Part model, mm, in its own coordinate system. Face numbers are marked on the shaded views. Coordinates: 2 decimals unless noted, no trailing zeros. Loops run counter-clockwise (first coordinate to the right, second up) from the corner with the lowest first, then second, coordinate; pieces in that order, holes last. Notation, with made-up numbers: (36, 10.5) - (44, 10.5) arc R14 ccw to (44, 25.5) - close; hole circle Ø11 at (-19, 80). An arc over 180 degrees is marked (long way). Use a Markdown table: item, result. Add a question column.
1. Band-saw the part on C-C, the plane x = 15.5. Give the cut face in (y, z).
2. Drop flat-ended pins along their axis: pin 1 (4 mm diameter, centred on x = 0, y = -9.5, fed in from -Z); pin 2 (5.5 mm diameter, centred on x = -15.5, y = 0, fed in from +Z); pin 3 (2 mm diameter, centred on x = -7.5, z = 2, fed in from +Y); pin 4 (1.5 mm diameter, centred on x = -5.5, z = 3, fed in from -Y). Give the stop position or say it passes through.
3. Band-saw the part on D-D, the plane x = -11. Give the cut face in (y, z).
4. Band-saw the part on B-B, the plane y = 0. Give the cut face in (x, z), plus the area to 3 significant figures.
5. Wall check: probe 1 along Y at (x, z) = (0, 1.2); probe 2 along Y at (x, z) = (0, 3.4); probe 3 along Z at (x, y) = (14, -1.5). Give the ranges that are in metal, low to high. Write a range as [from, to].
6. Pull direction X, two halves, no side cores. Call the marked faces 1, 2 and 3: pulls with the +X half, pulls with the -X half, needs draft (parallel to the pull), parting line crosses it, or undercut.
7. Band-saw the part on A-A, the plane z = 3.8. Give the cut face in (x, y), plus the area to 3 significant figures.
from build123d import *

# Parameters (mm, degrees)
F0_R     = 22.5
F1_DEPTH = 5
F3_DEPTH = 25
F5_DEPTH = 25
F6_R     = 2
F7_DEPTH = 25
F8_R     = 3.5
F9_DEPTH = 2.5


with BuildPart() as f1:
    # F0 (on Top) → F1 (new body)
    with BuildSketch(Plane.XY):
        Circle(F0_R)
    extrude(amount=F1_DEPTH)

    # F2 (on face) → F3 (cut)
    with BuildSketch(Plane.XY.offset(5)):
        with BuildLine():
            Line((2.7, 0), (2.7, 2.5298221281))
            ThreePointArc((2.7, 2.5298221281), (-3.7, 0), (2.7, -2.5298221281))
            Line((2.7, -2.5298221281), (2.7, 0))
        make_face()
    extrude(amount=-F3_DEPTH, mode=Mode.SUBTRACT)

    # F4 (on face) → F5 (cut)
    with BuildSketch(Plane.XY.offset(5)):
        with BuildLine():
            ThreePointArc((0, 17.5), (-1.4142135624, 14.0857864376), (2, 15.5))
            ThreePointArc((2, 15.5), (1.4142135624, 16.9142135624), (0, 17.5))
        make_face()
    extrude(amount=-F5_DEPTH, mode=Mode.SUBTRACT)

    # F6 (on face) → F7 (cut)
    with BuildSketch(Plane.XY.offset(5)):
        with Locations((15.5, 0)):
            Circle(F6_R)
        with BuildLine():
            ThreePointArc((0, -17.5), (1.4142135624, -16.9142135624), (2, -15.5))
            ThreePointArc((2, -15.5), (-1.4142135624, -14.0857864376), (0, -17.5))
        make_face()
        with BuildLine():
            ThreePointArc((-17.5, 0), (-15.5, -2), (-13.5, 0))
            ThreePointArc((-13.5, 0), (-15.5, 2), (-17.5, 0))
        make_face()
    extrude(amount=-F7_DEPTH, mode=Mode.SUBTRACT)

    # F8 (on face) → F9 (cut)
    with BuildSketch(Plane.XY.offset(5)):
        with Locations((-15.5, 0)):
            Circle(F8_R)
        with Locations((15.5, 0)):
            Circle(F8_R)
        with Locations((0, -15.5)):
            Circle(F8_R)
        with Locations((0, 15.5)):
            Circle(F8_R)
    extrude(amount=-F9_DEPTH, mode=Mode.SUBTRACT)


solid = f1.part
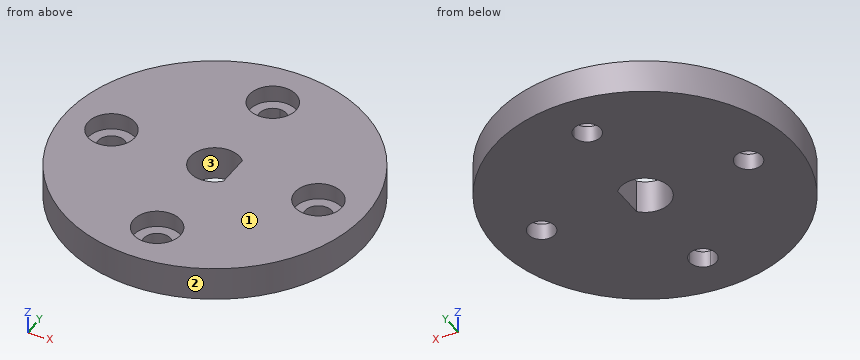
Geometry check:
| question | item | result |
|---|---|---|
| 1 | outline | (-16.31, 0) - (-2, 0) - (-2, 2.5) - (-3.5, 2.5) - (-3.5, 5) - (-16.31, 5) - close; (2, 0) - (16.31, 0) - (16.31, 5) - (3.5, 5) - (3.5, 2.5) - (2, 2.5) - close |
| 2 | pin 1 | stops at z = 0 |
| 2 | pin 2 | stops at z = 2.5 |
| 2 | pin 3 | stops at y = 21.54 |
| 2 | pin 4 | stops at y = -21.99 |
| 3 | outline | (-19.63, 0) - (19.63, 0) - (19.63, 5) - (-19.63, 5) - close |
| 4 | outline | (-22.5, 0) - (-17.5, 0) - (-17.5, 2.5) - (-19, 2.5) - (-19, 5) - (-22.5, 5) - close; (-13.5, 0) - (-3.7, 0) - (-3.7, 5) - (-12, 5) - (-12, 2.5) - (-13.5, 2.5) - close; (2.7, 0) - (13.5, 0) - (13.5, 2.5) - (12, 2.5) - (12, 5) - (2.7, 5) - close; (17.5, 0) - (22.5, 0) - (22.5, 5) - (19, 5) - (19, 2.5) - (17.5, 2.5) - close |
| 4 | area | 138 mm^2 |
| 5 | probe 1 | y = [-22.5, -17.5], [-13.5, -3.7], [3.7, 13.5], [17.5, 22.5] |
| 5 | probe 2 | y = [-22.5, -19], [-12, -3.7], [3.7, 12], [19, 22.5] |
| 5 | probe 3 | z = [0, 2.5] |
| 6 | face 1 | needs draft |
| 6 | face 2 | parting line crosses it |
| 6 | face 3 | undercut |
| 7 | outline | circle Ø45 at (0, 0); hole circle Ø7 at (-15.5, 0); hole circle Ø7 at (0, -15.5); hole circle Ø7 at (0, 15.5); hole (2.7, -2.53) - (2.7, 2.53) arc R3.7 ccw (long way) to start; hole circle Ø7 at (15.5, 0) |
| 7 | area | 1,400 mm^2 |
